from build123d import *

# Parameters (mm, degrees)
F0_W     = 74.732258
F0_H     = 60.57189
F1_DEPTH = 90
F2_R     = 4
F3_DEPTH = 90.001
F4_R     = 10


with BuildPart() as f1:
    # F0 (on Front) → F1 (new body)
    with BuildSketch(Plane.XZ):
        Rectangle(F0_W, F0_H)
    extrude(amount=F1_DEPTH)

    # F2 (on face) → F3 (cut, through all)
    with BuildSketch(Plane.XZ.offset(90)):
        Circle(F2_R)
    extrude(amount=-F3_DEPTH, mode=Mode.SUBTRACT)

    # F4
    f4_edges = [f1.edges().sort_by_distance(p)[0] for p in [
        (-37.366129, -90, 0),
        (37.366129, -90, 0),
        (0, -90, 30.285945),
        (-37.366129, -45, -30.285945),
        (37.366129, -45, -30.285945),
        (0, 0, -30.285945),
        (37.366129, -45, 30.285945),
        (37.366129, 0, 0),
        (-37.366129, -45, 30.285945),
        (-37.366129, 0, 0),
        (0, 0, 30.285945),
        (-4, -90, 0),
        (-4, 0, 0),
        (0, -90, -30.285945),
    ]]
    fillet(f4_edges, radius=F4_R)


solid = f1.part
Part model, mm, in its own coordinate system. Give positions to 0.01 mm unless a question says otherwise; leave off trailing zeros. Loops run counter-clockwise (first coordinate to the right, second up) from the corner with the lowest first, then second, coordinate; pieces in that order, holes last.
(1) Band-saw the part on B-B (x = 0). Write the cut outline in (y, z).
Return value:
outline: (-90, -20.29) arc R10 ccw to (-80, -30.29) - (-10, -30.29) arc R10 ccw to (0, -20.29) - (0, -14) arc R10 ccw to (-10, -4) - (-80, -4) arc R10 ccw to (-90, -14) - close; (-90, 14) arc R10 ccw to (-80, 4) - (-10, 4) arc R10 ccw to (0, 14) - (0, 20.29) arc R10 ccw to (-10, 30.29) - (-80, 30.29) arc R10 ccw to (-90, 20.29) - close
(2) Drill centre lines: line 1 along Z through (x, y) = (0, -33); line 2 along X through (y, z) = (-59, -1.5); line 3 along X through (y, z) = (-8.5, -1.5). Where is each one in solid material? Low to high.
Return value:
line 1: z = -30.29 to -4, 4 to 30.29
line 2: x = -37.37 to -3.71, 3.71 to 37.37
line 3: x = -37.25 to -3.83, 3.83 to 37.25
(3) Pin check, flat tip, straight feed: pin 1 (3 mm diameter, centred on x = -13.5, z = 22.5, fed in from -Y). Stop position of the tip, or through.
Return value:
pin 1: stops at y = -89.97
(4) Band-saw the part on A-A (z = 0). Write the cut outline in (x, y).
Return value:
outline: (-37.37, -80) arc R10 ccw to (-27.37, -90) - (-14, -90) arc R10 ccw to (-4, -80) - (-4, -10) arc R10 ccw to (-14, 0) - (-27.37, 0) arc R10 ccw to (-37.37, -10) - close; (4, -80) arc R10 ccw to (14, -90) - (27.37, -90) arc R10 ccw to (37.37, -80) - (37.37, -10) arc R10 ccw to (27.37, 0) - (14, 0) arc R10 ccw to (4, -10) - close
(5) Pull direction Z, two halves, no side cores. Call faces 1 (the cylindrical face through (-0.867, -45.49, -3.905)), 2 (the cylindrical face through (0.383, -86.993, -27.434)), 3 (the flat face through (0, -45, 30.286)), 4 (the cylindrical face through (-34.515, -86.993, 0.284)): pulls with the +Z half, pulls with the -Z half, needs draft (parallel to the pull), parting line crosses it, or undercut.
Return value:
face 1: undercut
face 2: pulls with the -Z half
face 3: pulls with the +Z half
face 4: needs draft
(6) Band-saw the part on D-D (x = 16.5). Write the cut outline in (y, z).
Return value:
outline: (-90, -20.29) arc R10 ccw to (-80, -30.29) - (-10, -30.29) arc R10 ccw to (0, -20.29) - (0, 20.29) arc R10 ccw to (-10, 30.29) - (-80, 30.29) arc R10 ccw to (-90, 20.29) - close
(7) Band-saw the part on C-C (y = -39.5). Write the cut outline in (x, z).
Return value:
outline: (-37.37, -20.29) arc R10 ccw to (-27.37, -30.29) - (27.37, -30.29) arc R10 ccw to (37.37, -20.29) - (37.37, 20.29) arc R10 ccw to (27.37, 30.29) - (-27.37, 30.29) arc R10 ccw to (-37.37, 20.29) - close; hole circle Ø8 at (0, 0)
